```python
from build123d import *

# Parameters (mm, degrees)
SKETCH1_R                    = 19.05
BOSS_EXTRUDE1_DEPTH          = 220.472
SKETCH2_R                    = 12.7
CUT_EXTRUDE1_DEPTH           = 221.472
F_1_1_4_7_TAPPED_HOLE1_D     = 28.17876
F_1_1_4_7_TAPPED_HOLE1_DEPTH = 49.022
F_1_1_4_7_TAPPED_HOLE1_TIP   = 8.465753589
F_1_1_4_7_TAPPED_HOLE2_D     = 28.17876
F_1_1_4_7_TAPPED_HOLE2_DEPTH = 49.022
F_1_1_4_7_TAPPED_HOLE2_TIP   = 8.465753589


with BuildPart() as part:
    # Sketch1 → Boss-Extrude1 (new body)
    with BuildSketch(Plane(origin=(0, 0, 0), x_dir=(1, 0, 0), z_dir=(0, 1, 0))):
        Circle(SKETCH1_R)
    extrude(amount=BOSS_EXTRUDE1_DEPTH)

    # Sketch2 → Cut-Extrude1 (cut, through all)
    with BuildSketch(Plane(origin=(0, 220.472, 0), x_dir=(1, 0, 0), z_dir=(0, 1, 0))):
        Circle(SKETCH2_R)
    extrude(amount=-CUT_EXTRUDE1_DEPTH, mode=Mode.SUBTRACT)

    # 1-1/4-7 Tapped Hole1
    with Locations(Plane(origin=(0, 220.472, 0), x_dir=(1, 0, 0), z_dir=(0, 1, 0))):
        with Locations((0, 0)):
            Hole(F_1_1_4_7_TAPPED_HOLE1_D / 2, depth=F_1_1_4_7_TAPPED_HOLE1_DEPTH)
            with Locations((0, 0, -(F_1_1_4_7_TAPPED_HOLE1_DEPTH + F_1_1_4_7_TAPPED_HOLE1_TIP / 2))):  # 118° drill point
                Cone(0, F_1_1_4_7_TAPPED_HOLE1_D / 2, F_1_1_4_7_TAPPED_HOLE1_TIP, mode=Mode.SUBTRACT)

    # 1-1/4-7 Tapped Hole2
    with Locations(Plane(origin=(0, 0, 0), x_dir=(-1, 0, 0), z_dir=(0, -1, 0))):
        with Locations((0, 0)):
            Hole(F_1_1_4_7_TAPPED_HOLE2_D / 2, depth=F_1_1_4_7_TAPPED_HOLE2_DEPTH)
            with Locations((0, 0, -(F_1_1_4_7_TAPPED_HOLE2_DEPTH + F_1_1_4_7_TAPPED_HOLE2_TIP / 2))):  # 118° drill point
                Cone(0, F_1_1_4_7_TAPPED_HOLE2_D / 2, F_1_1_4_7_TAPPED_HOLE2_TIP, mode=Mode.SUBTRACT)


solid = part.part
```
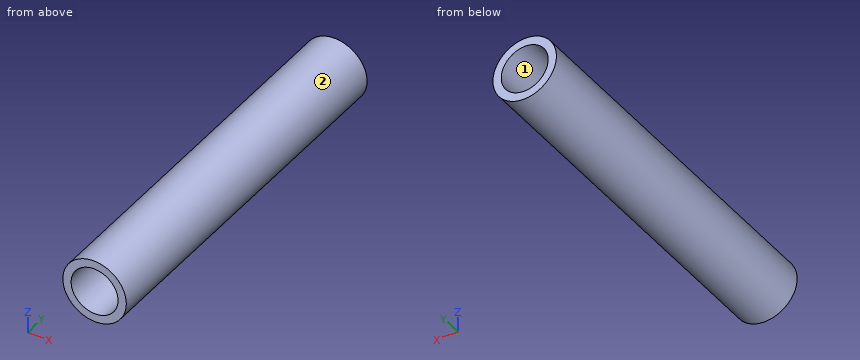
Read the model definition and answer for the solid it produces. Units are mm, in the model's axes. Face numbers are marked on the shaded views. Give positions to 0.01 mm unless a question says otherwise; leave off trailing zeros. Write each loop counter-clockwise with the first axis right and the second up, starting at its lowest first coordinate (ties: lowest second). Pieces come first, ordered by that corner, then holes. Notation, with made-up numbers: (29, 78.5) -> (69, 78.5) arc R35 cw to (69, 110.5) -> close; hole circle Ø11 at (35, 57). An arc over 180 degrees is marked (long way). Answer in a Markdown table with one row per item.
1) Section C-C on y = 137.5 is taken. Give the vertices of the cut face in (x, z), plus the area to 3 significant figures.
Results list:
| item | result |
|---|---|
| outline | circle Ø38.1 at (0, 0); hole circle Ø25.4 at (0, 0) |
| area | 633 mm^2 |
2) Section D-D on y = 179 is taken. Give the vertices of the cut face in (x, z), plus the area to 3 significant figures.
Results list:
| item | result |
|---|---|
| outline | circle Ø38.1 at (0, 0); hole circle Ø28.18 at (0, 0) |
| area | 516 mm^2 |
3) Straight lines are drawn through the part: line 1 (Z direction, x = 0, y = 111.5); line 2 (Z direction, x = 0, y = 191.5). For each, find the intervals that lie inside material, in ascending order. Write a range as [from, to].
Results list:
| item | result |
|---|---|
| line 1 | [-19.05, -12.7], [12.7, 19.05] |
| line 2 | [-19.05, -14.09], [14.09, 19.05] |
4) Section A-A on x = 0 is taken. Give the vertices of the cut face in (y, z).
Results list:
| item | result |
|---|---|
| outline | (0, -19.05) -> (220.47, -19.05) -> (220.47, -14.09) -> (171.45, -14.09) -> (170.62, -12.7) -> (49.86, -12.7) -> (49.02, -14.09) -> (0, -14.09) -> close; (0, 14.09) -> (49.02, 14.09) -> (49.86, 12.7) -> (170.62, 12.7) -> (171.45, 14.09) -> (220.47, 14.09) -> (220.47, 19.05) -> (0, 19.05) -> close |
5) Each of these flat-tipped pins is pushed along its axis until it touches: pin 1 Ø2 at (y, z) = (164, -14.5) entering from -X; pin 2 Ø2 at (x, y) = (-4, 34.5) entering from +Z; pin 3 Ø6 at (x, z) = (0.5, -11) entering from -Y; pin 4 Ø17 at (x, z) = (0, 0) entering from -Y. Where does it stop, or does it pass through?
Results list:
| item | result |
|---|---|
| pin 1 | x = -13.44 |
| pin 2 | z = 18.81 |
| pin 3 | y = 49.07 |
| pin 4 | through |
6) Determine the mould class of the marked faces 1 and 2 for opening direction X: released by +X, released by -X, zero draft, split by the parting line, or undercut.
Results list:
| item | result |
|---|---|
| face 1 | undercut |
| face 2 | split by the parting line |
7) Section B-B on z = 0 is taken. Give the vertices of the cut face in (x, y).
Results list:
| item | result |
|---|---|
| outline | (-19.05, 0) -> (-14.09, 0) -> (-14.09, 49.02) -> (-12.7, 49.86) -> (-12.7, 170.62) -> (-14.09, 171.45) -> (-14.09, 220.47) -> (-19.05, 220.47) -> close; (12.7, 49.86) -> (14.09, 49.02) -> (14.09, 0) -> (19.05, 0) -> (19.05, 220.47) -> (14.09, 220.47) -> (14.09, 171.45) -> (12.7, 170.62) -> close |
